Source: CAD feature listing. Evaluate the final solid. Frame: model axes, mm. A direction names the side the tool comes from. Give positions to 0.01 mm unless a question says otherwise; leave off trailing zeros. Write each loop counter-clockwise with the first axis right and the second up, starting at its lowest first coordinate (ties: lowest second). Pieces come first, ordered by that corner, then holes. Notation, with made-up numbers: (-20, -38.75) -> (-15, -38.75) arc R23 cw to (-15, -1.75) -> close; hole circle Ø1 at (60, -32). An arc over 180 degrees is marked (long way). Use one line per item in the form item = value. Start each with the question number.
(1) Draft query along Z for faces 4 (the face through (-5, 19, 3)), 5 (the face through (0, 21, 6.5)), 6 (the face through (7.76, 22.63, 3.38)). Return one class per face: pulls with the +Z half, pulls with the -Z half, needs draft (parallel to the pull), parting line crosses it, or undercut.
(2) Cut plane B-B, the plane z = 3.25. Output: boundary loops of the cut face in (x, y).
(3) Cut plane C-C, the plane y = 23.25. Output: boundary loops of the cut face in (x, z), and give its area (3 significant figures).
(4) Cut plane A-A, the plane x = 0. Output: boundary loops of the cut face in (y, z), and give its area (3 significant figures).
(5) Cut plane D-D, the plane y = 17.75. Output: boundary loops of the cut face in (x, z), and give its area (3 significant figures).
(6) Material intervals for line 1 along X through (y, z) = (22.6, 3.25); line 2 along Z through (x, y) = (8.75, 22.45); line 3 along X through (y, z) = (18.75, 1), sorted ascending. Write a range as from..to.
(7) First-contact query: P1, Ø1.8, axis at x = 8.75, z = 3.25, coming from the +Y side; P2, Ø3, axis at x = -8.5, z = 3, coming from the -Y side; P3, Ø1.3, axis at y = 18.5, z = 2.5, coming from the -X side; P4, Ø2, axis at y = 18.5, z = 2.5, coming from the +X side. Flat tips, straight axial feed; report the tip coordinate or a pass-through.
(8) Set-up query: faces 1 (the face through (-7, 21.363, 3)), 2 (the face through (7, 21.363, 3)), 3 (the face through (-10.43, 22.6, 0.6)). Return all of +Z, -Z, +X, -X, +Y, -Y with unobstructed straight access to the full face (end or side cutting, diameter ignored); none if empty.
from build123d import *

# Parameters (mm, degrees)
SKETCH1_W           = 10
SKETCH1_H           = 4
SKETCH1_R           = 1.5
SKETCH1_H_2         = 3
BOSS_EXTRUDE1_DEPTH = 6.5
SKETCH12_W          = 22
SKETCH12_H          = 6.5
SKETCH12_R          = 1
BOSS_EXTRUDE2_DEPTH = 2.5
FILLET1_R           = 2


with BuildPart() as part:
    # Sketch1 → Boss-Extrude1 (new body)
    # profile 1 of 2: a face of its own
    with BuildSketch(Plane.XY):
        with Locations((0, 18.863386012)):
            Rectangle(SKETCH1_W, SKETCH1_H)
        with Locations(Location((0, 18.863386012, 0), (0, 0, 180))):
            Circle(SKETCH1_R, mode=Mode.SUBTRACT)
    # profile 2 of 2: a face of its own
    with BuildSketch(Plane.XY):
        with Locations((0, 22.363386012)):
            Rectangle(SKETCH1_W, SKETCH1_H_2)
    extrude(amount=BOSS_EXTRUDE1_DEPTH)

    # Sketch12 → Boss-Extrude2 (add)
    with BuildSketch(Plane(origin=(0, 23.863386012, 0), x_dir=(1, 0, 0), z_dir=(0, 1, 0))):
        with Locations((0, -3.25)):
            Rectangle(SKETCH12_W, SKETCH12_H)
        with Locations(Location((-8.75, -3.25, 0), (0, 0, 270))):
            Circle(SKETCH12_R, mode=Mode.SUBTRACT)
        with Locations(Location((8.75, -3.25, 0), (0, 0, 90))):
            Circle(SKETCH12_R, mode=Mode.SUBTRACT)
    extrude(amount=-BOSS_EXTRUDE2_DEPTH)

    # Fillet1
    fillet1_edges = [part.edges().sort_by_distance(p)[0] for p in [
        (-11, 22.613386012, 0),
        (11, 22.613386012, 0),
        (11, 22.613386012, 6.5),
        (-11, 22.613386012, 6.5),
    ]]
    fillet(fillet1_edges, radius=FILLET1_R)


solid = part.part
Geometry says:
q1.face_4 = needs draft
q1.face_5 = pulls with the +Z half
q1.face_6 = undercut
q2.outline = (-11, 21.36) -> (-9.75, 21.36) -> (-9.75, 23.86) -> (-11, 23.86) -> close; (-7.75, 21.36) -> (-5, 21.36) -> (-5, 16.86) -> (5, 16.86) -> (5, 21.36) -> (7.75, 21.36) -> (7.75, 23.86) -> (-7.75, 23.86) -> close; (9.75, 21.36) -> (11, 21.36) -> (11, 23.86) -> (9.75, 23.86) -> close; hole circle Ø3 at (0, 18.86)
q3.outline = (-11, 2) arc R2 ccw to (-9, 0) -> (9, 0) arc R2 ccw to (11, 2) -> (11, 4.5) arc R2 ccw to (9, 6.5) -> (-9, 6.5) arc R2 ccw to (-11, 4.5) -> close; hole circle Ø2 at (-8.75, 3.25); hole circle Ø2 at (8.75, 3.25)
q3.area = 133 mm^2
q4.outline = (16.86, 0) -> (17.36, 0) -> (17.36, 6.5) -> (16.86, 6.5) -> close; (20.36, 0) -> (23.86, 0) -> (23.86, 6.5) -> (20.36, 6.5) -> close
q4.area = 26.0 mm^2
q5.outline = (-5, 0) -> (-1.01, 0) -> (-1.01, 6.5) -> (-5, 6.5) -> close; (1.01, 0) -> (5, 0) -> (5, 6.5) -> (1.01, 6.5) -> close
q5.area = 51.9 mm^2
q6.line_1 = -11..-9.75, -7.75..7.75, 9.75..11
q6.line_2 = 0..2.25, 4.25..6.5
q6.line_3 = -5..-1.5, 1.5..5
q7.P1 = through
q7.P2 = 21.36
q7.P3 = -5
q7.P4 = 5
q8.face_1 = +Z, -Z, -X, -Y
q8.face_2 = +Z, -Z, +X, -Y
q8.face_3 = -Z, -X, +Y, -Y
